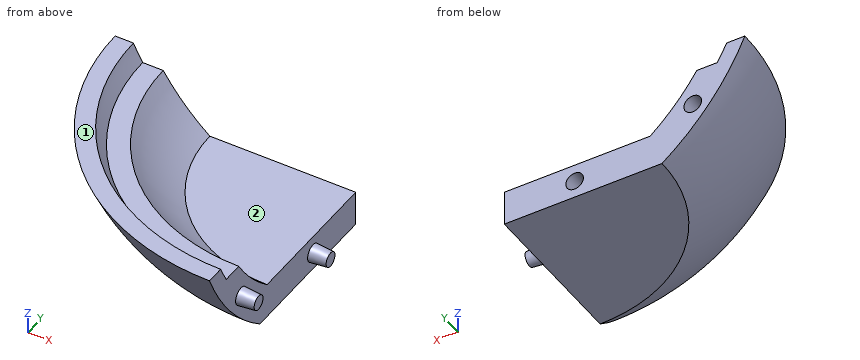
from build123d import *

# Parameters (mm, degrees)
F1_ANGLE = 90
F2_R     = 6.35
F3_DEPTH = 12.7
F3_TAPER = 5
F4_R     = 6.35
F5_DEPTH = 12.7
F5_TAPER = 5


with BuildPart() as f1:
    # F0 (on Front) → F1 (revolve)
    with BuildSketch(Plane.XZ):
        with BuildLine():
            ThreePointArc((-77.1013106813, -170.4810645103), (-80.5622641491, -164.1983062461), (-83.7669886019, -157.7810645103))
            Line((-83.7669886019, -157.7810645103), (-96.971668303, -157.7810645103))
            ThreePointArc((-96.971668303, -157.7810645103), (-71.9810472081, -199.7397034229), (-37.1588170528, -233.9810645103))
            Line((-37.1588170528, -233.9810645103), (76.7419968518, -233.9810645103))
            Line((76.7419968518, -233.9810645103), (76.7419968518, -208.5815945789))
            Line((76.7419968518, -208.5815945789), (-28.6076346844, -208.5815945789))
            ThreePointArc((-28.6076346844, -208.5815945789), (-46.9000470933, -190.8333294487), (-62.2427515075, -170.4810645103))
            Line((-62.2427515075, -170.4810645103), (-77.1013106813, -170.4810645103))
        make_face()
    revolve(axis=Axis((76.7419968518, 0, -221.2813295446), (0, 0, 1)), revolution_arc=F1_ANGLE)

    # F2 (on face) → F3 (join)
    with BuildSketch(Plane.YZ.offset(76.7419968518)):
        with Locations((-136.3420439451, -195.8810645103)):
            Circle(F2_R)
        with Locations((-50.7999999993, -221.2815945789)):
            Circle(F2_R)
    extrude(amount=F3_DEPTH, taper=F3_TAPER)

    # F4 (on face) → F5 (cut)
    with BuildSketch(Plane(origin=(0, 0, 0), x_dir=(-1, 0, 0), z_dir=(0, 1, 0))):
        with Locations((-25.9419968518, -221.2815945789)):
            Circle(F4_R)
        with Locations((59.3110422283, -195.8810645103)):
            Circle(F4_R)
    extrude(amount=-F5_DEPTH, taper=F5_TAPER, mode=Mode.SUBTRACT)


solid = f1.part
Can you work these out from the model? Positions are in its coordinate system, mm. Face numbers are marked on the shaded views. A direction names the side the tool comes from. Round coordinates to 2 decimals unless told otherwise and drop trailing zeros. Write each question's results on one line, items separated by ' | '. Start each with the question number.
Item 1: Will these pins go through, and if not, where does the flat tip stop? pin 1 (5 mm diameter, centred on x = -20.5, y = -85.5, fed in from +Z); pin 2 (2 mm diameter, centred on x = 20.5, z = -189, fed in from +Y); pin 3 (8 mm diameter, centred on x = -24, z = -167.5, fed in from +Y).
Item 2: Please list where these lines run through material, in increasing order: L1, parallel to Z at x = 36.5, y = -75; L2, parallel to Z at x = 67, y = -136; L3, parallel to X at y = -68.5, z = -189.5.
Item 3: Which directions (+Z, -Z, +X, -X, +Y, -Y) give clear straight access to the entire face, cutting with the end or side of a thin tool? Please do the marked faces 1 and 2.
Results:
1) pin 1: stops at z = -180.58 | pin 2: stops at y = -110.8 | pin 3: stops at y = -92.86
2) L1: z = -233.98 to -208.58 | L2: z = -213.99 to -174.48 | L3: x = -63.66 to -27.59
3) face 1: +Z, +X, -X, +Y, -Y | face 2: +Z, +X, +Y
